Input: part model. Units: mm. Frame: model coordinates. A direction names the side the tool comes from. Give positions to 0.01 mm unless a question says otherwise; leave off trailing zeros. Loops run counter-clockwise (first coordinate to the right, second up) from the corner with the lowest first, then second, coordinate; pieces in that order, holes last. Notation, with made-up numbers: M 33,11 L 56,11 A21 ccw 56,16 Z; hole C 64.5,17 d10. An arc over 180 degrees is marked long. Answer as a JSON object with one key per item and string values. Group by question number.
1) Section query B-B on z = 4.25. Return loops of the section in (x, y).
2) Section query C-C on y = 0. Return loops of the section in (x, z), plus the area to 3 significant figures.
3) Ray query, L1, parallel to Y at x = 0, z = 3; L2, parallel to Y at x = -6.5, z = 3.75; L3, parallel to X at y = 2, z = 6.75. Return the intervals inside material, ascending.
4) First-contact query: P1, Ø3, axis at x = -6.5, y = -6, coming from the +Z side; P2, Ø1.8, axis at y = 1, z = 4, coming from the -X side; P3, Ø4, axis at x = -21, z = 3.5, coming from the -Y side. Flat tips, straight axial feed; report the tip coordinate or a pass-through.
5) Access query for faces 4 (the flat face through (0, -11, 0)), 5 (the flat face through (22, 3, 4)), 6 (the flat face through (-22, 3, 4)). Directions: +Z, -Z, +X, -X, +Y, -Y. A direction counts if a zero-diameter tool reaches every point of the face in a straight line with its end or side. Return the directions, or none.
6) Section query A-A on x = 0. Return loops of the section in (y, z), plus the area to 3 significant figures.
7) Draft query along X for faces 1 (the flat face through (-22, -3, 4)), 2 (the conical face through (0.5, 24.63, 7.365)), 3 (the cylindrical face through (-2.17, -9.76, 3.7)). Return one class per face: +X half, -X half, draft (parallel to the pull), parting line (faces both ways), or undercut.
from build123d import *

# Parameters (mm, degrees)
F0_R     = 10
F1_DEPTH = 7.5
F2_SIZE  = 0.5


with BuildPart() as f1:
    # F0 (on Top) → F1 (new body)
    with BuildSketch(Plane.XY):
        with BuildLine():
            Line((20, 3), (24.819347, 3))
            ThreePointArc((24.819347, 3), (0, 25), (-24.819347, 3))
            Line((-24.819347, 3), (-20, 3))
            Line((-20, 3), (-20, -3))
            Line((-20, -3), (-24.819347, -3))
            ThreePointArc((-24.819347, -3), (0, -25), (24.819347, -3))
            Line((24.819347, -3), (20, -3))
            Line((20, -3), (20, 3))
        make_face()
        Circle(F0_R, mode=Mode.SUBTRACT)
    extrude(amount=F1_DEPTH)

    # F2
    f2_edges = [f1.edges().sort_by_distance(p)[0] for p in [
        (22.409674, 3, 7.5),
        (0, 25, 7.5),
        (-22.409674, 3, 7.5),
        (-20, 0, 7.5),
        (-22.409674, -3, 7.5),
        (0, -25, 7.5),
        (22.409674, -3, 7.5),
        (20, 0, 7.5),
        (-10, 0, 7.5),
        (22.409674, 3, 0),
        (0, 25, 0),
        (-22.409674, 3, 0),
        (-20, 0, 0),
        (-22.409674, -3, 0),
        (0, -25, 0),
        (22.409674, -3, 0),
        (20, 0, 0),
        (-10, 0, 0),
    ]]
    chamfer(f2_edges, length=F2_SIZE)


solid = f1.part
Output:
{
 "1": {"outline": "M -24.82,-3 A25 ccw 24.82,-3 L 20,-3 L 20,3 L 24.82,3 A25 ccw -24.82,3 L -20,3 L -20,-3 Z; hole C 0,0 d20"},
 "2": {"outline": "M -20,0.5 L -19.5,0 L -10.5,0 L -10,0.5 L -10,7 L -10.5,7.5 L -19.5,7.5 L -20,7 Z; M 10,0.5 L 10.5,0 L 19.5,0 L 20,0.5 L 20,7 L 19.5,7.5 L 10.5,7.5 L 10,7 Z", "area": "149 mm^2"},
 "3": {"L1": "y = -25 to -10, 10 to 25", "L2": "y = -24.14 to -7.6, 7.6 to 24.14", "L3": "x = -20 to -9.8, 9.8 to 20"},
 "4": {"P1": "stops at z = 7.35", "P2": "stops at x = -20", "P3": "stops at y = -16.25"},
 "5": {"face 4": "-Z, +X, -X, +Y, -Y", "face 5": "+Z, -Z, +X", "face 6": "+Z, -Z, -X"},
 "6": {"outline": "M -25,0.5 L -24.5,0 L -10.5,0 L -10,0.5 L -10,7 L -10.5,7.5 L -24.5,7.5 L -25,7 Z; M 10,0.5 L 10.5,0 L 24.5,0 L 25,0.5 L 25,7 L 24.5,7.5 L 10.5,7.5 L 10,7 Z", "area": "224 mm^2"},
 "7": {"face 1": "draft", "face 2": "parting line", "face 3": "undercut"}
}
